```python
from build123d import *

# Parameters (mm, degrees)
BOSS_EXTRUDE1_DEPTH = 3
BOSS_EXTRUDE2_DEPTH = 20


with BuildPart() as part:
    # Sketch1 → Boss-Extrude1 (new body)
    with BuildSketch(Plane.XY):
        with BuildLine():
            ThreePointArc((12.275451386, 39.110148544), (12.067880772, 33.648168724), (13.127719813, 28.28598164))
            ThreePointArc((13.127719813, 28.28598164), (-5.7809e-05, 26.00056132), (-13.127971261, 28.285201272))
            ThreePointArc((-13.127971261, 28.285201272), (-12.06796259, 33.647129894), (-12.275256819, 39.10889939))
            ThreePointArc((-12.275256819, 39.10889939), (0.000238569, 36.332719941), (12.275451386, 39.110148544))
        make_face()
    extrude(amount=BOSS_EXTRUDE1_DEPTH)

    # Sketch2 → Boss-Extrude2 (add)
    with BuildSketch(Plane(origin=(0, 0, 0), x_dir=(-1, 0, 0), z_dir=(0, 0, -1))):
        with BuildLine():
            ThreePointArc((-0.000238569, 33.482719941), (6.116423648, 34.084515432), (11.998357864, 35.867368305))
            ThreePointArc((11.998357864, 35.867368305), (12.080645356, 37.492931332), (12.275256819, 39.10889939))
            ThreePointArc((12.275256819, 39.10889939), (-0.000238569, 36.332719941), (-12.275451386, 39.110148544))
            ThreePointArc((-12.275451386, 39.110148544), (-12.080742195, 37.494064654), (-11.998373995, 35.868378864))
            ThreePointArc((-11.998373995, 35.868378864), (-6.116717522, 34.085055957), (-0.000238569, 33.482719941))
        make_face()
        with BuildLine():
            ThreePointArc((-13.127719813, 28.28598164), (5.7809e-05, 26.00056132), (13.127971261, 28.285201272))
            ThreePointArc((13.127971261, 28.285201272), (12.730383089, 29.661389101), (12.417381714, 31.059244398))
            ThreePointArc((12.417381714, 31.059244398), (5.905e-06, 28.850561321), (-12.417221823, 31.060076762))
            ThreePointArc((-12.417221823, 31.060076762), (-12.730176217, 29.662196758), (-13.127719813, 28.28598164))
        make_face()
    extrude(amount=BOSS_EXTRUDE2_DEPTH)


solid = part.part
```
Geometry: final body of the model. Coordinates: model frame, mm. A direction names the side the tool comes from. Coordinates: 2 decimals unless noted, no trailing zeros. Order: outer loops, then holes, each group sorted by start corner. A loop starts at its lowest first (then second) coordinate and runs counter-clockwise, first axis right, second up. Notation, with made-up numbers: (61.25, 89) - (65.25, 89) arc R29 ccw to (65.25, 122) - close; hole circle Ø6 at (82, 4.5). An arc over 180 degrees is marked (long way). Return JSON: item names as keys, results as strings. Group by question number.
1. Cut plane A-A (z = -3.5). Output: boundary loops of the cut face in (x, y), plus the area to 3 significant figures.
2. Pull-direction query (X, two-part tool) for faces 3 (the face through (-0.177, 36.333, -8.339)), 4 (the face through (0, 26, -9)), 5 (the face through (0, 33, 3)); classes: pulls with the +X half, pulls with the -X half, needs draft (parallel to the pull), parting line crosses it, or undercut.
3. Set-up query: faces 1 (the face through (0, 28, -20)), 2 (the face through (-0.18, 28.85, -9.86)). Return all of +Z, -Z, +X, -X, +Y, -Y with unobstructed straight access to the full face (end or side cutting, diameter ignored); none if empty.
4. Cut plane D-D (z = 1.5). Output: boundary loops of the cut face in (x, y), plus the area to 3 significant figures.
5. Pin query (flat end, axial travel): pin 1 (12 mm diameter, centred on x = -4, z = -13.5, fed in from +Y); pin 2 (4 mm diameter, centred on y = 30.5, z = -7, fed in from -X); pin 3 (12 mm diameter, centred on x = -1.5, z = -11.5, fed in from +Y). Return the tip coordinate at first contact, or that it passes through.
6. Cut plane C-C (y = 29.5). Output: boundary loops of the cut face in (x, z), plus the area to 3 significant figures.
7. Cut plane B-B (x = -8.75). Output: boundary loops of the cut face in (y, z), plus the area to 3 significant figures.
8. Material intervals for line 1 along Z through (x, y) = (-4.5, 30.5); line 2 along Y through (x, z) = (2.75, -8); line 3 along Y through (x, z) = (5.5, -1.25), sorted ascending. Write a range as [from, to].
Resolved:
{
 "1": {"outline": "(-13.13, 28.29) arc R38.85 ccw to (13.13, 28.29) arc R23.5 cw to (12.42, 31.06) arc R36 cw to (-12.42, 31.06) arc R23.5 cw to start; (-12.28, 39.11) arc R23.5 cw to (-12, 35.87) arc R31.37 ccw to (12, 35.87) arc R23.5 cw to (12.28, 39.11) arc R28.52 cw to start", "area": "145 mm²"},
 "2": {"face 3": "undercut", "face 4": "parting line crosses it", "face 5": "needs draft"},
 "3": {"face 1": "-Z, +X, -X, +Y, -Y", "face 2": "-Z"},
 "4": {"outline": "(-13.13, 28.29) arc R38.85 ccw to (13.13, 28.29) arc R23.5 cw to (12.28, 39.11) arc R28.52 cw to (-12.28, 39.11) arc R23.5 cw to start", "area": "260 mm²"},
 "5": {"pin 1": "stops at y = 38.14", "pin 2": "stops at x = -13.06", "pin 3": "stops at y = 37.34"},
 "6": {"outline": "(-12.77, -20) - (-6.81, -20) - (-6.81, 0) - (6.81, 0) - (6.81, -20) - (12.77, -20) - (12.77, 3) - (-12.77, 3) - close", "area": "315 mm²"},
 "7": {"outline": "(27, -20) - (29.93, -20) - (29.93, 0) - (34.73, 0) - (34.73, -20) - (37.71, -20) - (37.71, 3) - (27, 3) - close", "area": "150 mm²"},
 "8": {"line 1": "z = [0, 3]", "line 2": "y = [26.1, 28.96], [33.6, 36.47]", "line 3": "y = [26.39, 29.27], [33.97, 36.87]"}
}
